CAD build for the part. Positions are in the model's coordinates, mm. Coordinates: 2 decimals unless noted, no trailing zeros. Write each loop counter-clockwise with the first axis right and the second up, starting at its lowest first coordinate (ties: lowest second). Pieces come first, ordered by that corner, then holes. Notation, with made-up numbers: (84, 8.25) - (127, 8.25) arc R18 ccw to (127, 35.25) - close; hole circle Ø9 at (36.5, 25). An arc over 180 degrees is marked (long way). Answer in a Markdown table with one row per item. Add a question column.
Q1. Pin check, flat tips, straight feed: pin 1 (4 mm diameter, centred on x = 173.39, y = 15.17, fed in from +Z); pin 2 (1.5 mm diameter, centred on y = 87, z = 5.5, fed in from -X). Stop position of each tip, or through.
Q2. Band-saw the part on A-A (z = 3.25). State how many separate pieces and enclosed holes the cut face has, and give its area (3 significant figures).
Q3. Drill centre lines: line 1 along X through (y, z) = (-149.5, 2); line 2 along X through (y, z) = (-101, 3); line 3 along Y through (x, z) = (-14.5, 1.25). Where is each one in solid material? Low to high. Write a range as from..to.
Q4. Band-saw the part on B-B (x = -66.5). List the corners of the cut face in (y, z), and give its area (3 significant figures).
Q5. Two-plate mould, pull along X, no slides. Class faces 1 (the flat face through (38, 3, 0)), 2 (the cylindrical face through (1.38, -6.2, 3.13)), 3 (the cylindrical face through (-146.1, -112.1, 3.1)): +X half, -X half, draft (parallel to the pull), parting line (faces both ways), or undercut.
```python
from build123d import *

# Parameters (mm, degrees)
SKETCH2_R           = 184.15
BOSS_EXTRUDE1_DEPTH = 6.35
SKETCH9_R           = 2.38125
CUT_EXTRUDE4_DEPTH  = 261.504832009
CIRPATTERN1_COUNT   = 72
SKETCH10_R          = 6.35
CUT_EXTRUDE7_DEPTH  = 261.504832009


with BuildPart() as part:
    # Sketch2 → Boss-Extrude1 (new body)
    with BuildSketch(Plane.XY):
        Circle(SKETCH2_R)
    extrude(amount=BOSS_EXTRUDE1_DEPTH)

    # Sketch9 → Cut-Extrude4 (cut, through all)
    with BuildSketch(Plane.XY.offset(6.35)):
        with Locations((-174.049180881, 0)):
            Circle(SKETCH9_R)
    cut_extrude4 = extrude(amount=-CUT_EXTRUDE4_DEPTH, mode=Mode.SUBTRACT)

    # CirPattern1: Cut-Extrude4 ×72 about axis
    cirpattern1_axis = Axis((0, 0, 0), (0, 0, 1))
    for i in range(1, CIRPATTERN1_COUNT):
        add(cut_extrude4.rotate(cirpattern1_axis, i * 360 / CIRPATTERN1_COUNT), mode=Mode.SUBTRACT)

    # Sketch10 → Cut-Extrude7 (cut, through all)
    with BuildSketch(Plane(origin=(0, 0, 0), x_dir=(-1, 0, 0), z_dir=(0, 0, -1))):
        Circle(SKETCH10_R)
    extrude(amount=-CUT_EXTRUDE7_DEPTH, mode=Mode.SUBTRACT)


solid = part.part
```
Checked values:
| question | item | result |
|---|---|---|
| 1 | pin 1 | passes through |
| 1 | pin 2 | stops at x = -162.7 |
| 2 | separate pieces | 1 |
| 2 | enclosed holes | 73 |
| 2 | area | 105,000 mm² |
| 3 | line 1 | x = -107.52..-89.06, -84.99..84.99, 89.06..107.52 |
| 3 | line 2 | x = -153.98..-144.65, -140.5..140.5, 144.65..153.98 |
| 3 | line 3 | y = -183.58..-175.67, -171.1..171.1, 175.67..183.58 |
| 4 | outline | (-171.72, 0) - (171.72, 0) - (171.72, 6.35) - (-171.72, 6.35) - close |
| 4 | area | 2,180 mm² |
| 5 | face 1 | draft |
| 5 | face 2 | undercut |
| 5 | face 3 | parting line |
